Geometry check sheet. Reference: the model listing, model coordinates, mm. Face numbers are marked on the shaded views. A direction names the side the tool comes from. Give positions to 0.01 mm unless a question says otherwise; leave off trailing zeros. Loops run counter-clockwise (first coordinate to the right, second up) from the corner with the lowest first, then second, coordinate; pieces in that order, holes last. Notation, with made-up numbers: (-37.5, 40.5) - (-28.5, 40.5) arc R20 cw to (-28.5, 59.5) - close; hole circle Ø4 at (75.5, -37.75). An arc over 180 degrees is marked (long way). One line per question, with ' | ' between items. Start each with the question number.
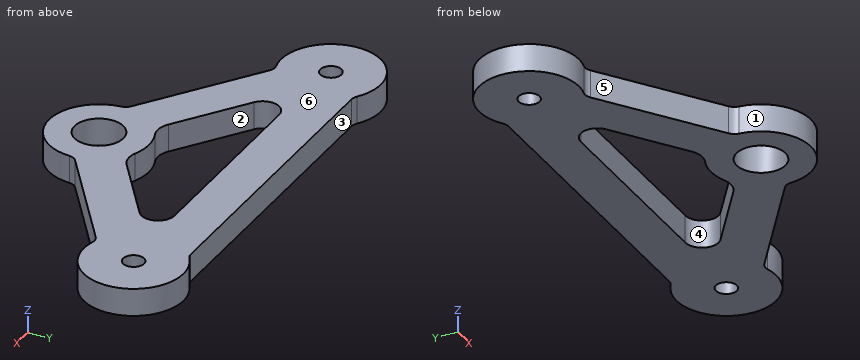
from build123d import *

# Parameters (mm, degrees)
ESQUISSE1_R        = 1.9
ESQUISSE1_R_2      = 4.4
BOSS_EXTRU_1_DEPTH = 5


with BuildPart() as part:
    # Esquisse1 → Boss.-Extru.1 (new body)
    with BuildSketch(Plane.XY):
        with BuildLine():
            Line((30.300082727, 2.968924298), (9.763004104, -11.338457247))
            ThreePointArc((9.763004104, -11.338457247), (9.172405802, -11.982601165), (8.912853429, -12.817083223))
            ThreePointArc((8.912853429, -12.817083223), (-0.078877501, -21.086221809), (-9.031083885, -12.77430994))
            ThreePointArc((-9.031083885, -12.77430994), (-9.286654991, -11.938599972), (-9.874175684, -11.291647751))
            Line((-9.874175684, -11.291647751), (-30.342811787, 3.113479848))
            ThreePointArc((-30.342811787, 3.113479848), (-31.150105491, 3.448150462), (-32.023034153, 3.406640278))
            ThreePointArc((-32.023034153, 3.406640278), (-43.269038369, 13.640318644), (-29.212114116, 19.437185406))
            ThreePointArc((-29.212114116, 19.437185406), (-28.66359268, 19.164598239), (-28.058297671, 19.070803357))
            Line((-28.058297671, 19.070803357), (28.299854, 19.070803357))
            ThreePointArc((28.299854, 19.070803357), (28.91331959, 19.167212023), (29.467641782, 19.447143388))
            ThreePointArc((29.467641782, 19.447143388), (43.297743059, 13.302630265), (31.981683615, 3.25407109))
            ThreePointArc((31.981683615, 3.25407109), (31.108962768, 3.29974241), (30.300082727, 2.968924298))
        make_face()
        with Locations((-34.404288116, 12.085904623)):
            Circle(ESQUISSE1_R, mode=Mode.SUBTRACT)
        with Locations((34.404288116, 11.921884391)):
            Circle(ESQUISSE1_R, mode=Mode.SUBTRACT)
        with Locations((-0.057424101, -12.086247379)):
            Circle(ESQUISSE1_R_2, mode=Mode.SUBTRACT)
        with BuildLine():
            Line((-18.288536611, 11.047420606), (18.173688409, 11.047420606))
            ThreePointArc((18.173688409, 11.047420606), (21.194925395, 8.966949346), (19.94448595, 5.518379385))
            Line((19.94448595, 5.518379385), (7.224114855, -3.343407178))
            ThreePointArc((7.224114855, -3.343407178), (5.36635505, -4.038296984), (3.403177648, -3.755316724))
            ThreePointArc((3.403177648, -3.755316724), (-0.06139684, -3.06515242), (-3.525362111, -3.758367937))
            ThreePointArc((-3.525362111, -3.758367937), (-5.489866285, -4.031985712), (-7.344292156, -3.328247102))
            Line((-7.344292156, -3.328247102), (-20.022270936, 5.59408196))
            ThreePointArc((-20.022270936, 5.59408196), (-21.154680468, 8.956364593), (-18.288536611, 11.047420606))
        make_face(mode=Mode.SUBTRACT)
    extrude(amount=BOSS_EXTRU_1_DEPTH)


solid = part.part
(1) Depth check by flat-ended pin: pin 1 Ø11.5 at (x, y) = (-0.06, -12.09) entering from -Z; pin 2 Ø1.5 at (x, z) = (19.5, 3.5) entering from -Y; pin 3 Ø1.5 at (y, z) = (-6, 2.5) entering from -X. Enter the tip coordinate at first touch or a pass-through.
(2) Section check C-C, the plane z = 4.05. Record the boundary of the cut face in (x, y).
(3) Mould release check, pull along X, two halves, no side actions. Record for the marked faces 4, 5 and 6: pulls with the +X half, pulls with the -X half, needs draft (parallel to the pull), parting line crosses it, or undercut.
(4) Material ranges on line 1 (X direction, y = -1, z = 1); line 2 (X direction, y = 13, z = 1.6); line 3 (X direction, y = 5.5, z = 0.75), recorded low to high.
(5) Section check D-D, the plane y = -8.5. Record the boundary of the cut face in (x, z), and give its area (3 significant figures).
(6) Section check A-A, the plane y = 0.5. Record the boundary of the cut face in (x, z), and give its area (3 significant figures).
(7) Section check B-B, the plane x = 0. Record the boundary of the cut face in (y, z).
(8) Tool access check on the marked faces 1, 2 and 3. Record the directions out of +Z, -Z, +X, -X, +Y, -Y that give a thin tool (end or side, any length) a straight path to the whole face; none if there is none.
Numbers:
1) pin 1: z = 0 | pin 2: y = -5.08 | pin 3: x = -18.46
2) outline: (-32.02, 3.41) arc R2 cw to (-30.34, 3.11) - (-9.87, -11.29) arc R2 cw to (-9.03, -12.77) arc R9 ccw to (8.91, -12.82) arc R2 cw to (9.76, -11.34) - (30.3, 2.97) arc R2 cw to (31.98, 3.25) arc R9 ccw (long way) to (29.47, 19.45) arc R2 cw to (28.3, 19.07) - (-28.06, 19.07) arc R2 cw to (-29.21, 19.44) arc R9 ccw (long way) to start; hole circle Ø3.8 at (-34.4, 12.09); hole (-20.02, 5.59) - (-7.34, -3.33) arc R4 ccw to (-3.53, -3.76) arc R9.02 cw to (3.4, -3.76) arc R4 ccw to (7.22, -3.34) - (19.94, 5.52) arc R3 ccw to (18.17, 11.05) - (-18.29, 11.05) arc R3 ccw to start; hole circle Ø8.8 at (-0.06, -12.09); hole circle Ø3.8 at (34.4, 11.92)
3) face 4: undercut | face 5: pulls with the -X half | face 6: needs draft
4) line 1: -24.5 to -10.65, 10.59 to 24.6 | line 2: -43.36 to -36.07, -32.74 to 32.84, 35.97 to 43.34 | line 3: -40.54 to -19.89, 19.92 to 40.71
5) outline: (-13.84, 0) - (-2.61, 0) - (-2.61, 5) - (-13.84, 5) - close; (2.49, 0) - (13.84, 0) - (13.84, 5) - (2.49, 5) - close | area: 113 mm^2
6) outline: (-26.63, 0) - (-12.78, 0) - (-12.78, 5) - (-26.63, 5) - close; (12.74, 0) - (26.76, 0) - (26.76, 5) - (12.74, 5) - close | area: 139 mm^2
7) outline: (-21.09, 0) - (-16.49, 0) - (-16.49, 5) - (-21.09, 5) - close; (-7.69, 0) - (-3.07, 0) - (-3.07, 5) - (-7.69, 5) - close; (11.05, 0) - (19.07, 0) - (19.07, 5) - (11.05, 5) - close
8) face 1: +Z, -Z, -Y | face 2: +Z, -Z | face 3: +Z, -Z, +Y
